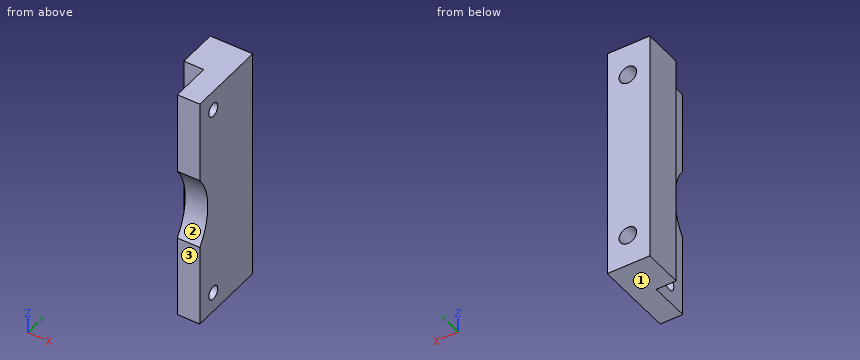
from build123d import *

# Parameters (mm, degrees)
F4_R      = 5
F5_DEPTH  = 17
F7_W      = 30
F7_H      = 178
F8_DEPTH  = 15
F10_D     = 10.2
F10_DEPTH = 80
F10_START = 31
F10_TIP   = 3.064389157
F11_D     = 13.2
F11_DEPTH = 30
F11_TIP   = 3.9656800856


with BuildPart() as f5:
    # F4 (on offset) → F5 (new body)
    with BuildSketch(Plane.YZ.offset(-48)):
        with BuildLine():
            Line((36, 89), (36, 27))
            ThreePointArc((36, 27), (45, 0), (36, -27))
            Line((36, -27), (36, -89))
            Line((36, -89), (96, -89))
            Line((96, -89), (96, 89))
            Line((96, 89), (36, 89))
        make_face()
        with Locations((51.2249938995, -74)):
            Circle(F4_R, mode=Mode.SUBTRACT)
        with Locations((51.2249938995, 74)):
            Circle(F4_R, mode=Mode.SUBTRACT)
        with Locations((51.2249938995, 74)):
            Circle(F4_R)
        with Locations((51.2249938995, -74)):
            Circle(F4_R)
    extrude(amount=F5_DEPTH)

    # F7 (on face) → F8 (join)
    with BuildSketch(Plane(origin=(-48, 0, 0), x_dir=(0, -1, 0), z_dir=(-1, 0, 0))):
        with Locations((-81, 0)):
            Rectangle(F7_W, F7_H)
    extrude(amount=F8_DEPTH)

    # F10
    # its depths count from where the whole tool has entered the part; down to there all is cleared
    with Locations(Plane.YZ.offset(-F10_START)):
        with Locations((51.2249938995, 74), (51.2249938995, -74)):
            Hole(F10_D / 2, depth=F10_DEPTH)
            with Locations((0, 0, -(F10_DEPTH + F10_TIP / 2))):  # 118° drill point
                Cone(0, F10_D / 2, F10_TIP, mode=Mode.SUBTRACT)

    # F11
    with Locations(Plane(origin=(0, 96, 0), x_dir=(-1, 0, 0), z_dir=(0, 1, 0))):
        with Locations((46.5, 65), (46.5, -65)):
            Hole(F11_D / 2, depth=F11_DEPTH)
            with Locations((0, 0, -(F11_DEPTH + F11_TIP / 2))):  # 118° drill point
                Cone(0, F11_D / 2, F11_TIP, mode=Mode.SUBTRACT)


solid = f5.part
Part model, mm, in its own coordinate system. Face numbers are marked on the shaded views. Give positions to 0.01 mm unless a question says otherwise; leave off trailing zeros. Loops run counter-clockwise (first coordinate to the right, second up) from the corner with the lowest first, then second, coordinate; pieces in that order, holes last. Notation, with made-up numbers: (87.5, 85.25) -> (125.5, 85.25) arc R13 ccw to (125.5, 90.25) -> close; hole circle Ø10 at (21, 12.25). An arc over 180 degrees is marked (long way). Write each question's results on one line, items separated by ' | '. Start each with the question number.
Q1. Wall check: L1, parallel to Z at x = -46, y = 84.5; L2, parallel to Z at x = -33.5, y = 55; L3, parallel to Y at x = -56.5, z = -54. Give the ranges that are in metal, low to high.
Q2. Pin check, flat tips, straight feed: P1, Ø4, axis at y = 57.5, z = 44.5, coming from the -X side; P2, Ø10, axis at x = -47.5, z = 64, coming from the +Y side; P3, Ø7.5, axis at x = -54.5, z = 23, coming from the -Y side. Stop position of each tip, or through.
Q3. Band-saw the part on B-B on y = 54. List the corners of the cut face in (x, z), plus the area to 3 significant figures.
Q4. Pull direction Z, two halves, no side cores. Call the marked faces 1, 2 and 3: +Z half, -Z half, draft (parallel to the pull), parting line (faces both ways), or undercut.
Q5. Band-saw the part on D-D on z = -46.5. List the corners of the cut face in (x, y), plus the area to 3 significant figures.
Q6. Band-saw the part on A-A on z = 74. List the corners of the cut face in (x, y) (3 decimals), plus the area to 3 significant figures.
Q7. Band-saw the part on C-C on y = 69. List the corners of the cut face in (x, z), plus the area to 3 significant figures.
Results are:
1) L1: z = -89 to -71.58, -58.42 to 58.42, 71.58 to 89 | L2: z = -89 to -77.43, -70.57 to 70.57, 77.43 to 89 | L3: y = 66 to 96
2) P1: stops at x = -48 | P2: stops at y = 65.74 | P3: stops at y = 66
3) outline: (-48, -89) -> (-31, -89) -> (-31, -78.28) -> (-48, -78.28) -> close; (-48, -69.72) -> (-31, -69.72) -> (-31, 69.72) -> (-48, 69.72) -> close; (-48, 78.28) -> (-31, 78.28) -> (-31, 89) -> (-48, 89) -> close | area: 2,740 mm²
4) face 1: -Z half | face 2: undercut | face 3: draft
5) outline: (-63, 66) -> (-48, 66) -> (-48, 36) -> (-31, 36) -> (-31, 96) -> (-63, 96) -> close | area: 1,470 mm²
6) outline: (-63, 66) -> (-48, 66) -> (-48, 56.325) -> (-31, 56.325) -> (-31, 96) -> (-63, 96) -> close; (-48, 36) -> (-31, 36) -> (-31, 46.125) -> (-48, 46.125) -> close | area: 1,300 mm²
7) outline: (-63, -89) -> (-31, -89) -> (-31, 89) -> (-63, 89) -> close; hole circle Ø13.2 at (-46.5, -65); hole circle Ø13.2 at (-46.5, 65) | area: 5,420 mm²
